Autodesk Inventor part; units mm, degrees
ref_plane "YZ Plane" through (0, 0, 0) normal (1, 0, 0) x (0, 1, 0)
ref_plane "XZ Plane" through (0, 0, 0) normal (0, 1, 0) x (-1, 0, 0)
ref_plane "XY Plane" through (0, 0, 0) normal (0, 0, 1) x (1, 0, 0)
sketch "Sketch1" plane through (0, 0, 0) normal (0, 0, 1) x (1, 0, 0)
  line L0 (0, 0) -> (0, 136.525) construction
  line L1 (-11.7886, 12.2907) -> (-39.6863, 18.4755) construction
  line L2 (-39.6863, 18.4755) -> (-33.3297, 47.1481) construction
  line L3 (-33.3297, 47.1481) -> (-5.432, 40.9633) construction
  line L4 (-5.432, 40.9633) -> (-11.7886, 12.2907) construction
  line L5 (-39.6863, 18.4755) -> (-5.432, 40.9633) construction
  line L6 (-33.3297, 47.1481) -> (-11.7886, 12.2907) construction
  circle A0 centre (-53.975, 12.7) radius 3.175 construction
  circle A1 centre (-53.975, 12.7) radius 6.35 construction
  line L7 (0, 0) -> (-54.712, 6.3929) construction
  line L8 (-59.6703, 15.5082) -> (0, 136.525) construction
  line L9 (-27.1302, 45.7737) -> (-37.4529, 28.5497) construction
  line L10 (-11.6315, 42.3377) -> (-9.5552, 22.3649) construction
  line L11 (-19.3809, 44.0557) -> (-25.7374, 15.3831) construction
  line L12 (0, 92.075) -> (-19.7574, 96.4551) construction
  line L13 (-35.3766, 8.5768) -> (-19.8779, 5.1408) construction
  line L14 (-19.8779, 5.1408) -> (-21.2523, -1.0586) construction
  line L15 (-21.2523, -1.0586) -> (-36.751, 2.3773) construction
  line L16 (-36.751, 2.3773) -> (-35.3766, 8.5768) construction
  line L17 (-35.3766, 8.5768) -> (-41.27, 4.8223) construction
  line L18 (-19.8779, 5.1408) -> (-17.9381, 2.096) construction
  line L19 (-5.432, 40.9633) -> (-33.3297, 47.1481) construction
  line L20 (-33.3297, 47.1481) -> (-32.2475, 52.0296) construction
  line L21 (-32.2475, 52.0296) -> (-4.3498, 45.8448) construction
  line L22 (-4.3498, 45.8448) -> (-5.432, 40.9633) construction
  line L23 (-53.2878, 15.7997) -> (-53.975, 12.7) construction
  line L24 (-53.975, 12.7) -> (-57.0747, 13.3872) construction
  line L25 (-27.6272, 6.8588) -> (-34.4992, -24.1386) construction
  line L26 (-31.8676, 50.076) -> (-5.5198, 44.2349)
  line L27 (-5.5198, 44.2349) -> (-4.489, 48.8845) construction
  line L28 (-4.489, 48.8845) -> (-30.8368, 54.7256) construction
  line L29 (-30.8368, 54.7256) -> (-31.8676, 50.076) construction
  line L30 (-31.3522, 52.4008) -> (-5.0044, 46.5597) construction
  circle A2 centre (-29.0274, 51.8854) radius 1.4732 construction
  circle A3 centre (-22.8279, 50.5111) radius 1.4732 construction
  circle A4 centre (-16.6284, 49.1367) radius 1.4732 construction
  circle A5 centre (-10.4289, 47.7623) radius 1.4732
  circle A6 centre (-10.3614, 84.7398) radius 1.4732 construction
  line L31 (-53.975, 12.7) -> (-13.3751, 95.0402) construction
  line L32 (-32.2923, 56.6744) -> (0, 49.5153) construction
  circle A7 centre (-10.3614, 84.7398) radius 4.7625 construction
  line L33 (-4.7625, 50.5712) -> (-4.7625, 93.1308) construction
  line L34 (-27.5056, 55.6132) -> (-14.3936, 82.2055) construction
  line L35 (-5.6003, 84.6261) -> (-4.7625, 84.4403) construction
  line L36 (-17.9381, 2.096) -> (0, 2.096) construction
  line L37 (0, 2.096) -> (0, -1.079) construction
  line L38 (0, -1.079) -> (-17.9381, -1.079) construction
  line L39 (-17.9381, -1.079) -> (-17.9381, 2.096) construction
  circle A8 centre (-12.7, 7.9375) radius 1.5875 construction
  line L40 (-12.7, 7.9375) -> (0, 7.9375)
  line L41 (0, 7.9375) -> (-17.9381, 2.096) construction
  circle A9 centre (-12.7, 7.9375) radius 3.175 construction
  line L42 (-9.525, 7.9375) -> (-9.525, 4.8357) construction
  line L43 (-9.525, 7.9375) -> (0, 7.9375) construction
  line L44 (-17.9187, 46.9837) -> (-16.8879, 51.6333)
  line L45 (-12.4942, 45.7811) -> (-26.2381, -16.2137)
  line L46 (0, 66.675) -> (0, 7.9375)
  line L47 (-26.2381, -16.2137) -> (-20.0386, -17.5881)
  line L48 (-20.0386, -17.5881) -> (-8.7313, 7.9375)
  circle A10 centre (-12.7, 6.35) radius 1.4224
  line L49 (0, 13.4938) -> (-4.7625, 13.4938) construction
  line L50 (-4.7625, 13.4938) -> (-4.7625, 24.6063) construction
  line L51 (-4.7625, 24.6063) -> (0, 24.6063) construction
  line L52 (0, 24.6063) -> (0, 13.4938)
  line L53 (-4.7625, 19.05) -> (0, 19.05) construction
  circle A11 centre (-2.3813, 19.05) radius 1.4224
  line L54 (-20.7405, 8.5842) -> (-9.7454, 58.18)
  line L55 (-9.7454, 58.18) -> (-3.5459, 56.8056) construction
  line L56 (-3.5459, 56.8056) -> (-14.5411, 7.2098) construction
  line L57 (-14.5411, 7.2098) -> (-20.7405, 8.5842)
  line L58 (-12.7, 6.35) -> (-12.7, 7.9375) construction
  line L59 (-11.5442, 1.5875) -> (-9.525, 1.5875)
  line L60 (-9.525, 1.5875) -> (-9.525, 7.9375)
  line L61 (-9.525, 7.9375) -> (-11.5442, 7.9375)
  line L62 (-11.5442, 7.9375) -> (-11.5442, 1.5875) construction
  line L63 (-9.7454, 58.18) -> (-15.9449, 59.5544)
  line L64 (-15.9449, 59.5544) -> (-14.6504, 65.3933)
  line L65 (-14.6504, 65.3933) -> (0, 66.675)
  line L66 (-9.7454, 58.18) -> (-17.3193, 53.3549) construction
  arc A12 (-10.2313, 55.9882) -> (-11.9373, 58.6659) centre (-11.0843, 57.3271) ccw
  line L67 (-4.7625, 57.15) -> (0, 57.15) construction
  circle A13 centre (-2.3813, 57.15) radius 1.4224
  circle A14 centre (-2.3813, 63.5) radius 1.4224
  point P0 (-22.5591, 29.7194)
  point P1 (-20.4869, 2.3938)
  point P2 (-36.3367, 4.2458)
  point P3 (-51.1668, 18.3953)
  point P4 (-11.1125, 7.9375)
  point P5 (-11.4283, 6.9872)
  point P6 (-11.9574, 7.9375)
  point P7 (-13.9717, 6.9872)
  point P8 (-9.525, 6.1457)
  dimension "d74" = 6.35
  dimension "d13" = 136.525
  dimension "d14" = 29.3687
  dimension "d15" = 28.575
  dimension "d16" = 12.5
  dimension "d17" = 6.35
  dimension "d19" = 53.975
  dimension "d22" = 12.7
  dimension "d23" = 7.9375
  dimension "d24" = 19.05
  dimension "d26" = 102.5
  dimension "d29" = 6.35
  dimension "d31" = 7.9375
  dimension "d34" = 5
  dimension "d35" = 26.9875
  dimension "d38" = 31.75
  dimension "d40" = 26.9875
  dimension "d41" = 4.7625
  dimension "d42" = 2.9464
  dimension "d43" = 2.3813
  dimension "d46" = 6.35
  dimension "d51" = 2.9464
  dimension "d52" = 79.7719
  dimension "d53" = 6.35
  dimension "d54" = 9.525
  dimension "d55" = 4.7625
  dimension "d56" = 4.7625
  dimension "d60" = 12.7
  dimension "d61" = 3.175
  dimension "d63" = 3.175
  dimension "d66" = 3.175
  dimension "d67" = 12.7
  dimension "d72" = 8.7312
  dimension "d73" = 7.9375
  dimension "d75" = 34.925
  dimension "d80" = 12.7
  dimension "d82" = 7.9375
  dimension "d83" = 63.5
  dimension "d84" = 66.675
  dimension "d85" = 6.35
  dimension "d86" = 92.075
  dimension "d87" = 2.8448
  dimension "d88" = 4.7625
  dimension "d89" = 11.1125
  dimension "d90" = 2.8448
  dimension "d91" = 19.05
  dimension "d92" = 6.35
  dimension "d93" = 50.8
  dimension "d94" = 25.4
  dimension "d95" = 8.7312
  dimension "d96" = 9.525
  dimension "d97" = 6.35
  dimension "d99" = 6.35
  dimension "d101" = 3.175
  dimension "d106" = 2.8448
  dimension "d107" = 57.15
  dimension "d110" = 6.35
  dimension "d119" = 85
extrude "Extrusion1" add sketch "Sketch1" along normal blind 6.35 contours A5 | L60 L48 L47 L45 L54 A12 L63 L64 L65 L46 L40 | L40 L48 L60 | L60 L59 L48
fillet "Fillet1" radius 1.5875 8 edges at (-26.2381, -16.2137, 3.175) (-20.0386, -17.5881, 3.175) (-11.5442, 1.5875, 3.175) (-9.525, 1.5875, 3.175) (-14.6504, 65.3933, 3.175) (0, 66.675, 3.175) (-9.525, 6.1457, 3.175) (-8.7313, 7.9375, 3.175)
fillet "Fillet4" radius 1.5875 2 edges at (-10.2313, 55.9882, 3.175) (-11.9373, 58.6659, 3.175)
sketch "Sketch2" plane through (-15.9449, 59.5544, 0) normal (-0.2164396, -0.976296, 0) x (0.976296, -0.2164396, 0)
  line L0 (12.3735, 0) -> (1.1101, 0)
  line L1 (3.175, 0) -> (3.175, 6.35) construction
  line L2 (0, 6.35) -> (3.5733, 6.35)
  circle A0 centre (3.175, 3.175) radius 2.125
  line L3 (0, 0) -> (0, 6.35)
  point P0 (28.4569, 0)
  dimension "d115" = 4.25
  dimension "d116" = 3.175
extrude "Extrusion2" cut sketch "Sketch2" against normal through all
equation "\"d56\" = d55"
properties part number "Uprights" material "UHMW, White"
Read the model definition and answer for the solid it produces. Units are mm, in the model's axes. A direction names the side the tool comes from. Coordinates: 2 decimals unless noted, no trailing zeros. Order: outer loops, then holes, each group sorted by start corner. A loop starts at its lowest first (then second) coordinate and runs counter-clockwise, first axis right, second up. Notation, with made-up numbers: (5.25, 50) - (26.25, 50) arc R9 cw to (26.25, 54) - close; hole circle Ø11 at (46, -20.5). An arc over 180 degrees is marked (long way). Answer as a JSON object with one key per item and string values. Group by question number.
Item 1: Flat-ended cylindrical pins translate along their axes: P1, Ø2.5, axis at x = -2.38, y = 19.05, coming from the -Z side; P2, Ø1.9, axis at x = -2.5, z = 3.5, coming from the -Y side; P3, Ø0.8, axis at y = 4.5, z = 2, coming from the +X side (3 decimals). Find the tip coordinate at first contact, or state that the pin passes through.
Item 2: Section A-A (x = -3) is taken. Give the vertices of the cut face in (y, z), plus the area to 3 significant figures.
Item 3: A tool of negligible diameter and unlimited length cuts with its end or side. For faces 1 (the face through (-14.951, 59.334, 2.425)), 2 (the face through (-13.829, 7.216, 3.131)), 3 (the face through (-4, 7.938, 3)), from which of +Z, -Z, +X, -X, +Y, -Y can it reach the whole face along a straight path? Write none if from no direction.
Item 4: Section D-D (y = -2) is taken. Give the vertices of the cut face in (x, z).
Item 5: The mould has two halves that part along Y. Classify faces 4 (the face through (-10.1, 62.1, 2.4)), 5 (the face through (-9.525, 4, 3)), 6 (the face through (-0.5, 66.1, 3.2)), 7 (the face through (-20.3, -17.2, 3.2)): +Y half, -Y half, draft (parallel to the pull), parting line (faces both ways), or undercut.
Item 6: Consider probe 1 along Y at (x, z) = (-1.5, 3); probe 2 along Y at (x, z) = (-1.75, 1.25); probe 3 along X at (y, z) = (27, 2.75). Determine where each line is inside the solid, lowest interval first. Write a range as from..to.
Item 7: Section B-B (y = 19.05) is taken. Give the vertices of the cut face in (x, z), plus the area to 3 significant figures.
Item 8: Section C-C (y = 57.15) is taken. Give the vertices of the cut face in (x, z), plus the area to 3 significant figures.
Results are:
{
 "1": {"P1": "passes through", "P2": "stops at y = 7.94", "P3": "stops at x = -9.525"},
 "2": {"outline": "(7.94, 0) - (17.77, 0) - (17.77, 6.35) - (7.94, 6.35) - close; (20.33, 0) - (55.87, 0) - (55.87, 6.35) - (20.33, 6.35) - close; (58.43, 0) - (62.22, 0) - (62.22, 6.35) - (58.43, 6.35) - close; (64.78, 0) - (66.41, 0) - (66.41, 6.35) - (64.78, 6.35) - close", "area": "323 mm^2"},
 "3": {"face 1": "+Z, -Z, -X", "face 2": "+Z, -Z", "face 3": "+Z, -Z, +X, -Y"},
 "4": {"outline": "(-23.09, 0) - (-13.13, 0) - (-13.13, 6.35) - (-23.09, 6.35) - close"},
 "5": {"face 4": "undercut", "face 5": "draft", "face 6": "+Y half", "face 7": "-Y half"},
 "6": {"probe 1": "y = 7.94..17.93, 20.17..56.03, 58.27..62.38, 64.62..66.53", "probe 2": "y = 7.94..17.78, 20.32..55.88, 58.42..62.23, 64.77..66.52", "probe 3": "x = -16.66..0"},
 "7": {"outline": "(-18.42, 0) - (-3.8, 0) - (-3.8, 6.35) - (-18.42, 6.35) - close; (-0.96, 0) - (0, 0) - (0, 6.35) - (-0.96, 6.35) - close", "area": "98.9 mm^2"},
 "8": {"outline": "(-9.51, 0) - (-3.8, 0) - (-3.8, 6.35) - (-9.51, 6.35) - close; (-0.96, 0) - (0, 0) - (0, 6.35) - (-0.96, 6.35) - close", "area": "42.3 mm^2"}
}
